Design review of the part shown in the three views and the two pictorial views. Dimensions are in mm from the part's minimum x, y and z. A direction names the side the tool comes from. Round coordinates to 2 decimals unless told otherwise and drop trailing zeros. Loops run counter-clockwise (first coordinate to the right, second up) from the corner with the lowest first, then second, coordinate; pieces in that order, holes last. Notation, with made-up numbers: (25.25, 15.5) -> (40.25, 15.5) arc R18 cw to (40.25, 23.5) -> close; hole circle Ø7 at (82.25, -27). An arc over 180 degrees is marked (long way). Write each question's results on one line, items separated by ' | '. Start each with the question number.
Item 1: Mouldability with a two-part tool opening along X and no side actions: class the marked faces 5, 6 and 7 as pulls with the +X half, pulls with the -X half, needs draft (parallel to the pull), parting line crosses it, or undercut.
Item 2: Clearance check with flat-ended pins moving along their axes: pin 1 Ø2.5 at (x, y) = (2.5, 15.5) entering from +Z; pin 2 Ø3.5 at (x, z) = (4, 13) entering from -Y; pin 3 Ø6 at (y, z) = (4.5, 14.5) entering from +X. State where each tip first meets the part, or that it passes through.
Item 3: Tool access review of the marked faces 1, 2, 3 and 4: name each direction out of +Z, -Z, +X, -X, +Y, -Y from which nothing blocks a thin tool from reaching the whole face with its end or side.
Item 4: For L1, parallel to Z at x = 4, y = 15.45; L2, parallel to Z at x = 4.5, y = 16; L3, parallel to X at y = 12.5, z = 6.25, list the stretches that pass through material, from the lowest coordinate up. Write a range as from..to.
Item 5: We need section B-B (z = 7). Give the boundary of the cut face in (x, y), and give its area (3 significant figures).
Item 6: We need section D-D (z = 10.25). Give the boundary of the cut face in (x, y), and give its area (3 significant figures).
Item 7: We need section C-C (y = 16). Give the boundary of the cut face in (x, z), and give its area (3 significant figures).
Item 8: We need section A-A (x = 48). Give the boundary of the cut face in (y, z), and give its area (3 significant figures).
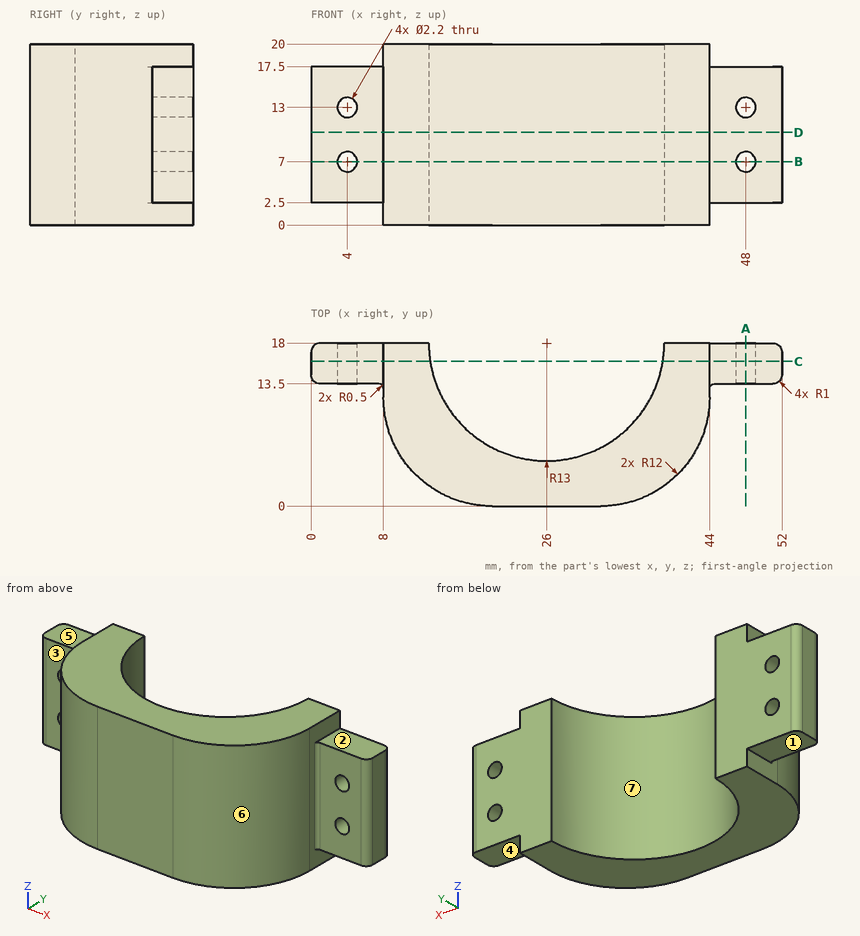
Here are the results:
1) face 5: needs draft | face 6: pulls with the +X half | face 7: undercut
2) pin 1: stops at z = 17.5 | pin 2: stops at y = 13.5 | pin 3: stops at x = 43.12
3) face 1: -Z, -X, +Y, -Y | face 2: +Z, +X, +Y, -Y | face 3: +Z, -Z, -X, -Y | face 4: -Z, +X, +Y, -Y
4) L1: z = 2.5..5.9, 8.1..11.9, 14.1..17.5 | L2: z = 2.5..6.02, 7.98..12.02, 13.98..17.5 | L3: x = 8..14.22, 37.78..44
5) outline: (0, 14.5) arc R1 ccw to (1, 13.5) -> (2.9, 13.5) -> (2.9, 18) -> (1, 18) arc R1 ccw to (0, 17) -> close; (5.1, 13.5) -> (7.5, 13.5) arc R0.5 cw to (8, 13) -> (8, 12) arc R12 ccw to (20, 0) -> (32, 0) arc R12 ccw to (44, 12) -> (44, 13) arc R0.5 cw to (44.5, 13.5) -> (46.9, 13.5) -> (46.9, 18) -> (39, 18) arc R13 cw to (13, 18) -> (5.1, 18) -> close; (49.1, 13.5) -> (51, 13.5) arc R1 ccw to (52, 14.5) -> (52, 17) arc R1 ccw to (51, 18) -> (49.1, 18) -> close | area: 372 mm2
6) outline: (0, 14.5) arc R1 ccw to (1, 13.5) -> (7.5, 13.5) arc R0.5 cw to (8, 13) -> (8, 12) arc R12 ccw to (20, 0) -> (32, 0) arc R12 ccw to (44, 12) -> (44, 13) arc R0.5 cw to (44.5, 13.5) -> (51, 13.5) arc R1 ccw to (52, 14.5) -> (52, 17) arc R1 ccw to (51, 18) -> (39, 18) arc R13 cw to (13, 18) -> (1, 18) arc R1 ccw to (0, 17) -> close | area: 392 mm2
7) outline: (0, 2.5) -> (8, 2.5) -> (8, 0) -> (13.15, 0) -> (13.15, 20) -> (8, 20) -> (8, 17.5) -> (0, 17.5) -> close; (38.85, 0) -> (44, 0) -> (44, 2.5) -> (52, 2.5) -> (52, 17.5) -> (44, 17.5) -> (44, 20) -> (38.85, 20) -> close; hole circle Ø2.2 at (4, 7); hole circle Ø2.2 at (4, 13); hole circle Ø2.2 at (48, 7); hole circle Ø2.2 at (48, 13) | area: 431 mm2
8) outline: (13.5, 2.5) -> (18, 2.5) -> (18, 5.9) -> (13.5, 5.9) -> close; (13.5, 8.1) -> (18, 8.1) -> (18, 11.9) -> (13.5, 11.9) -> close; (13.5, 14.1) -> (18, 14.1) -> (18, 17.5) -> (13.5, 17.5) -> close | area: 47.7 mm2
